```python
from build123d import *

# Parameters (mm, degrees)
SKETCH1_W           = 47.8
SKETCH1_H           = 10.8
BOSS_EXTRUDE1_DEPTH = 0.8
CUT_EXTRUDE1_REACH  = 26.516
SKETCH2_R           = 4.25
FILLET1_R           = 4.9


with BuildPart() as part:
    # Sketch1 → Boss-Extrude1 (new body)
    with BuildSketch(Plane(origin=(0, 0, 0), x_dir=(1, 0, 0), z_dir=(0, 1, 0))):
        Rectangle(SKETCH1_W, SKETCH1_H)
    extrude(amount=BOSS_EXTRUDE1_DEPTH)

    # Sketch2 → Cut-Extrude1 (cut, up to next)
    with BuildSketch(Plane(origin=(0, 0.8, 0), x_dir=(1, 0, 0), z_dir=(0, 1, 0)), mode=Mode.PRIVATE) as cut_extrude1_sk1:
        with Locations(Location((-18, 0, 0), (0, 0, 270))):
            Circle(SKETCH2_R)
    cut_extrude1_tool1 = extrude(cut_extrude1_sk1.sketch, amount=-CUT_EXTRUDE1_REACH, mode=Mode.PRIVATE) & part.part
    # Sketch2 → Cut-Extrude1 (cut, up to next)
    with BuildSketch(Plane(origin=(0, 0.8, 0), x_dir=(1, 0, 0), z_dir=(0, 1, 0)), mode=Mode.PRIVATE) as cut_extrude1_sk2:
        with Locations(Location((18, 0, 0), (0, 0, 270))):
            Circle(SKETCH2_R)
    cut_extrude1_tool2 = extrude(cut_extrude1_sk2.sketch, amount=-CUT_EXTRUDE1_REACH, mode=Mode.PRIVATE) & part.part
    # Sketch2 → Cut-Extrude1 (cut, up to next)
    with BuildSketch(Plane(origin=(0, 0.8, 0), x_dir=(1, 0, 0), z_dir=(0, 1, 0)), mode=Mode.PRIVATE) as cut_extrude1_sk3:
        with Locations(Location((-6, 0, 0), (0, 0, 270))):
            Circle(SKETCH2_R)
    cut_extrude1_tool3 = extrude(cut_extrude1_sk3.sketch, amount=-CUT_EXTRUDE1_REACH, mode=Mode.PRIVATE) & part.part
    # Sketch2 → Cut-Extrude1 (cut, up to next)
    with BuildSketch(Plane(origin=(0, 0.8, 0), x_dir=(1, 0, 0), z_dir=(0, 1, 0)), mode=Mode.PRIVATE) as cut_extrude1_sk4:
        with Locations(Location((6, 0, 0), (0, 0, 270))):
            Circle(SKETCH2_R)
    cut_extrude1_tool4 = extrude(cut_extrude1_sk4.sketch, amount=-CUT_EXTRUDE1_REACH, mode=Mode.PRIVATE) & part.part
    add(cut_extrude1_tool1.solids().sort_by_distance((-18, 0.8, 0))[0], mode=Mode.SUBTRACT)
    add(cut_extrude1_tool2.solids().sort_by_distance((18, 0.8, 0))[0], mode=Mode.SUBTRACT)
    add(cut_extrude1_tool3.solids().sort_by_distance((-6, 0.8, 0))[0], mode=Mode.SUBTRACT)
    add(cut_extrude1_tool4.solids().sort_by_distance((6, 0.8, 0))[0], mode=Mode.SUBTRACT)

    # Fillet1
    fillet1_edges = [part.edges().sort_by_distance(p)[0] for p in [
        (-23.9, 0.4, -5.4),
        (23.9, 0.4, -5.4),
        (23.9, 0.4, 5.4),
        (-23.9, 0.4, 5.4),
    ]]
    fillet(fillet1_edges, radius=FILLET1_R)


solid = part.part
```
Geometry check sheet. Reference: the model listing, model coordinates, mm. Give positions to 0.01 mm unless a question says otherwise; leave off trailing zeros. Order: outer loops, then holes, each group sorted by start corner. A loop starts at its lowest first (then second) coordinate and runs counter-clockwise, first axis right, second up. Notation, with made-up numbers: (35.5, 54.25) - (39.5, 54.25) arc R15 ccw to (39.5, 79.25) - close; hole circle Ø1 at (37, 70). An arc over 180 degrees is marked (long way). Answer in a Markdown table with one row per item. Add a question column.
Q1. Gauge pin test, flat end, axial feed: pin 1 (2 mm diameter, centred on x = 15, z = -3.5, fed in from -Y). Record the tip position at first contact, or that the pin passes through.
Q2. Cross-section at C-C, the plane x = -6. Enter the section's corners in (y, z).
Q3. Material ranges on probe 1 along X at (y, z) = (0.45, 0); probe 2 along X at (y, z) = (0.1, -2.25); probe 3 along Z at (x, y) = (3.5, 0.45), recorded low to high. Write a range as from..to.
Q4. Cross-section at D-D, the plane z = -1.75. Enter the section's corners in (x, y), then the cut area to 3 significant figures.
Q5. Cross-section at B-B, the plane z = 1.25. Enter the section's corners in (x, y).
Q6. Cross-section at A-A, the plane y = 0.45. Enter the section's corners in (x, z), then the cut area to 3 significant figures.
Q7. Mould release check, pull along X, two halves, no side actions. Record for faces 1 (the flat face through (0, 0.8, 0)), 2 (the cylindrical face through (-22.15, 0.41, -0.92)), 3 (the cylindrical face through (22.43, 0.41, -4)): pulls with the +X half, pulls with the -X half, needs draft (parallel to the pull), parting line crosses it, or undercut.
Check values:
| question | item | result |
|---|---|---|
| 1 | pin 1 | stops at y = 0 |
| 2 | outline | (0, -5.4) - (0.8, -5.4) - (0.8, -4.25) - (0, -4.25) - close; (0, 4.25) - (0.8, 4.25) - (0.8, 5.4) - (0, 5.4) - close |
| 3 | probe 1 | x = -23.9..-22.25, -13.75..-10.25, -1.75..1.75, 10.25..13.75, 22.25..23.9 |
| 3 | probe 2 | x = -23.58..-21.61, -14.39..-9.61, -2.39..2.39, 9.61..14.39, 21.61..23.58 |
| 3 | probe 3 | z = -5.4..-3.44, 3.44..5.4 |
| 4 | outline | (-23.74, 0) - (-21.87, 0) - (-21.87, 0.8) - (-23.74, 0.8) - close; (-14.13, 0) - (-9.87, 0) - (-9.87, 0.8) - (-14.13, 0.8) - close; (-2.13, 0) - (2.13, 0) - (2.13, 0.8) - (-2.13, 0.8) - close; (9.87, 0) - (14.13, 0) - (14.13, 0.8) - (9.87, 0.8) - close; (21.87, 0) - (23.74, 0) - (23.74, 0.8) - (21.87, 0.8) - close |
| 4 | area | 13.2 mm^2 |
| 5 | outline | (-23.84, 0) - (-22.06, 0) - (-22.06, 0.8) - (-23.84, 0.8) - close; (-13.94, 0) - (-10.06, 0) - (-10.06, 0.8) - (-13.94, 0.8) - close; (-1.94, 0) - (1.94, 0) - (1.94, 0.8) - (-1.94, 0.8) - close; (10.06, 0) - (13.94, 0) - (13.94, 0.8) - (10.06, 0.8) - close; (22.06, 0) - (23.84, 0) - (23.84, 0.8) - (22.06, 0.8) - close |
| 6 | outline | (-23.9, -0.5) arc R4.9 ccw to (-19, -5.4) - (19, -5.4) arc R4.9 ccw to (23.9, -0.5) - (23.9, 0.5) arc R4.9 ccw to (19, 5.4) - (-19, 5.4) arc R4.9 ccw to (-23.9, 0.5) - close; hole circle Ø8.5 at (-18, 0); hole circle Ø8.5 at (-6, 0); hole circle Ø8.5 at (6, 0); hole circle Ø8.5 at (18, 0) |
| 6 | area | 269 mm^2 |
| 7 | face 1 | needs draft |
| 7 | face 2 | undercut |
| 7 | face 3 | pulls with the +X half |
